from build123d import *

# Parameters (mm, degrees)
SKETCH1_R           = 3
BOSS_EXTRUDE1_DEPTH = 2
BOSS_EXTRUDE2_DEPTH = 4
CHAMFER1_SIZE       = 3
FILLET1_R           = 5


with BuildPart() as part:
    # Sketch1 → Boss-Extrude1 (new body)
    with BuildSketch(Plane.XY):
        with BuildLine():
            Line((24, -20), (-24, -20))
            Line((-24, -20), (-24, 20))
            Line((-24, 20), (-7, 20))
            Line((-7, 20), (-7, 29))
            ThreePointArc((-7, 29), (-5.535533906, 32.535533906), (-2, 34))
            Line((-2, 34), (2, 34))
            ThreePointArc((2, 34), (5.535533906, 32.535533906), (7, 29))
            Line((7, 29), (7, 20))
            Line((7, 20), (24, 20))
            Line((24, 20), (24, -20))
        make_face()
        with Locations((0, 28.5)):
            Circle(SKETCH1_R, mode=Mode.SUBTRACT)
    extrude(amount=BOSS_EXTRUDE1_DEPTH)

    # Sketch2 → Boss-Extrude2 (add)
    with BuildSketch(Plane.XY.offset(2)):
        Polygon((-22.5, -17.5), (-22.5, -19.10035342), (-0.5, -19.10035342), (-0.5, -17.5), (-0.5, 17.5), (-22.5, 17.5), align=None)
        Polygon((22.5, -17.5), (22.5, 17.5), (0.5, 17.5), (0.5, -17.5), (0.5, -19.10035342), (22.5, -19.10035342), align=None)
    extrude(amount=BOSS_EXTRUDE2_DEPTH)

    # Chamfer1
    chamfer1_edges = [part.edges().sort_by_distance(p)[0] for p in [
        (-22.5, 17.5, 4),
        (-22.5, -19.10035342, 4),
        (22.5, -19.10035342, 4),
        (22.5, 17.5, 4),
    ]]
    chamfer(chamfer1_edges, length=CHAMFER1_SIZE)

    # Fillet1
    fillet1_edges = [part.edges().sort_by_distance(p)[0] for p in [
        (-7, 20, 1),
        (7, 20, 1),
        (24, 20, 1),
        (24, -20, 1),
        (-24, -20, 1),
        (-24, 20, 1),
    ]]
    fillet(fillet1_edges, radius=FILLET1_R)


solid = part.part
Geometry: final body of the model. Coordinates: model frame, mm. A direction names the side the tool comes from. Round coordinates to 2 decimals unless told otherwise and drop trailing zeros. Order: outer loops, then holes, each group sorted by start corner. A loop starts at its lowest first (then second) coordinate and runs counter-clockwise, first axis right, second up. Notation, with made-up numbers: (-36.5, -31) -> (-25.5, -31) arc R28 cw to (-25.5, -7) -> close; hole circle Ø7 at (73.5, 18). An arc over 180 degrees is marked (long way). Put each result on its own line as item: value. Start each with the question number.
Q1. Section B-B on z = 0.85. Return the cut outline in (x, y).
Q2. Section A-A on z = 4.35. Return the cut outline in (x, y).
Q3. Line query: probe 1 along X at (y, z) = (-6, 4.55); probe 2 along Y at (x, z) = (0, 0.45); probe 3 along Y at (x, z) = (-2.5, 2.85). Output: solid intervals per line, ascending.
Q4. Reachability of faces 1 (the flat face through (21, -17.6, 4)), 2 (the flat face through (-0.5, -1, 4)), 3 (the flat face through (10, 17.5, 4)) from +Z, -Z, +X, -X, +Y, -Y: full face, straight path, thin tool, end or side. Return the list, or none.
Q5. First-contact query: pin 1 (1.2 mm diameter, centred on y = -1.5, z = 4, fed in from -X); pin 2 (0.6 mm diameter, centred on x = -16, z = 0.5, fed in from +Y); pin 3 (3 mm diameter, centred on x = 3.5, z = 5.5, fed in from -Y); pin 4 (5.5 mm diameter, centred on x = 0, y = 28.5, fed in from -Z). Flat tips, straight axial feed; report the tip coordinate or a pass-through.
Q6. Section D-D on y = 26.5. Return the cut outline in (x, z), and give its area (3 significant figures).
Q7. Section C-C on x = -16. Return the cut outline in (y, z), and give its area (3 significant figures).
Ans:
1. outline: (-24, -15) arc R5 ccw to (-19, -20) -> (19, -20) arc R5 ccw to (24, -15) -> (24, 15) arc R5 ccw to (19, 20) -> (12, 20) arc R5 cw to (7, 25) -> (7, 29) arc R5 ccw to (2, 34) -> (-2, 34) arc R5 ccw to (-7, 29) -> (-7, 25) arc R5 cw to (-12, 20) -> (-19, 20) arc R5 ccw to (-24, 15) -> close; hole circle Ø6 at (0, 28.5)
2. outline: (-22.5, -16.1) -> (-19.5, -19.1) -> (-0.5, -19.1) -> (-0.5, 17.5) -> (-19.5, 17.5) -> (-22.5, 14.5) -> close; (0.5, -19.1) -> (19.5, -19.1) -> (22.5, -16.1) -> (22.5, 14.5) -> (19.5, 17.5) -> (0.5, 17.5) -> close
3. probe 1: x = -22.5 to -0.5, 0.5 to 22.5
3. probe 2: y = -20 to 25.5, 31.5 to 34
3. probe 3: y = -19.1 to 17.5
4. face 1: +Z, +X, -Y
4. face 2: +Z, +Y, -Y
4. face 3: +Z, +X, -X, +Y
5. pin 1: stops at x = -22.5
5. pin 2: stops at y = 20
5. pin 3: stops at y = -19.1
5. pin 4: passes through
6. outline: (-7, 0) -> (-2.24, 0) -> (-2.24, 2) -> (-7, 2) -> close; (2.24, 0) -> (7, 0) -> (7, 2) -> (2.24, 2) -> close
6. area: 19.1 mm2
7. outline: (-20, 0) -> (20, 0) -> (20, 2) -> (17.5, 2) -> (17.5, 6) -> (-19.1, 6) -> (-19.1, 2) -> (-20, 2) -> close
7. area: 226 mm2
